from build123d import *

# Parameters (mm, degrees)
SKETCH_1_W            = 42.6
SKETCH_1_H            = 42.6
EXTRUDE_1_DEPTH       = 4
SKETCH_2_R            = 13
CUT_EXTRUDE_1_DEPTH   = 6
FILLET_1_R            = 10
SKETCH_3_W            = 4
SKETCH_3_H            = 22.6
EXTRUDE_2_DEPTH       = 34.5
FILLET_2_R            = 10
SKETCH_4_W            = 12
SKETCH_4_H            = 22.6
EXTRUDE_3_DEPTH       = 6
FILLET_3_R            = 5
FILLET_4_R            = 1
CHAMFER_3_SIZE        = 1
SKETCH_5_R            = 2.5
CUT_EXTRUDE_2_DEPTH   = 56.092921505
CHAMFER_START         = -9.101924
CHAMFER_4_DEPTH       = 6.602294476
CHAMFER_START_2       = 2.5000001
CHAMFER_4_2_DEPTH     = 6.6019239
CHAMFER_START_3       = -2.499629524
CHAMFER_4_3_DEPTH     = 4.999629624
CHAMFER_START_4       = -11.3
CHAMFER_4_4_DEPTH     = 2.198076
CHAMFER_START_5       = 9.101924
CHAMFER_4_5_DEPTH     = 2.198076
CHAMFER_START_6       = 16.5
CHAMFER_4_6_OUTLINE_R = 2.5
CHAMFER_4_6_DEPTH     = 12
SKETCH_6_R            = 4.2
CUT_EXTRUDE_5_DEPTH   = 28


with BuildPart() as part:
    # Эскиз1 → Бобышка-Вытянуть1 (new body)
    with BuildSketch(Plane(origin=(0, 0, 0), x_dir=(1, 0, 0), z_dir=(0, 1, 0))):
        Rectangle(SKETCH_1_W, SKETCH_1_H)
    extrude(amount=EXTRUDE_1_DEPTH)

    # Эскиз2 → Вырез-Вытянуть1 (cut)
    with BuildSketch(Plane(origin=(0, 4, 0), x_dir=(1, 0, 0), z_dir=(0, 1, 0))):
        with Locations(Location((0, 0, 0), (0, 0, 270))):
            Circle(SKETCH_2_R)
    extrude(amount=-CUT_EXTRUDE_1_DEPTH, mode=Mode.SUBTRACT)

    # Скругление1
    fillet_1_edges = [part.edges().sort_by_distance(p)[0] for p in [
        (21.3, 2, 21.3),
        (-21.3, 2, 21.3),
        (-21.3, 2, -21.3),
        (21.3, 2, -21.3),
    ]]
    fillet(fillet_1_edges, radius=FILLET_1_R)

    # Эскиз3 → Бобышка-Вытянуть2 (add)
    with BuildSketch(Plane(origin=(0, 0, 0), x_dir=(1, 0, 0), z_dir=(0, 1, 0))):
        with Locations((-23.3, 0)):
            Rectangle(SKETCH_3_W, SKETCH_3_H)
        with Locations((23.3, 0)):
            Rectangle(SKETCH_3_W, SKETCH_3_H)
    extrude(amount=EXTRUDE_2_DEPTH)

    # Скругление2
    # the kernel refuses this fillet: 10 mm, written as the material it adds along each edge
    with BuildSketch(Plane(origin=(21.3, 0, -11.3), x_dir=(-0.23904572186687842, 0, -0.9710083124552246), z_dir=(0, 1, 0)), Plane(origin=(-21.3, 0, 11.3), x_dir=(0.2390457218668792, 0, 0.9710083124552243), z_dir=(0, 1, 0))) as fillet_2_piece_1:
        with BuildLine():
            CenterArc((7.171371656, -9.710083125), FILLET_2_R, 103.83022495, 40.535802111)
            Line((-0.956182887, -3.88403325), (0, 0))
            ThreePointArc((0, 0), (2.390457219, -0.289916875), (4.780914437, 0))
        make_face()
    extrude(amount=4)
    with BuildSketch(Plane(origin=(-21.3, 0, -11.3), x_dir=(0.23904572186687842, 0, -0.9710083124552246), z_dir=(0, 1, 0)), Plane(origin=(21.3, 0, 11.3), x_dir=(-0.2390457218668792, 0, 0.9710083124552243), z_dir=(0, 1, 0))) as fillet_2_piece_2:
        with BuildLine():
            CenterArc((7.171371656, 9.710083125), FILLET_2_R, 215.633972939, 40.535802111)
            Line((-0.956182887, 3.88403325), (0, 0))
            ThreePointArc((0, 0), (2.390457219, 0.289916875), (4.780914437, 0))
        make_face()
    extrude(amount=4)

    # Эскиз4 → Бобышка-Вытянуть3 (add)
    with BuildSketch(Plane(origin=(0, 34.5, 0), x_dir=(1, 0, 0), z_dir=(0, 1, 0))):
        with Locations((-31.3, 0)):
            Rectangle(SKETCH_4_W, SKETCH_4_H)
        with Locations((31.3, 0)):
            Rectangle(SKETCH_4_W, SKETCH_4_H)
    extrude(amount=-EXTRUDE_3_DEPTH)

    # Скругление3
    fillet_3_edges = [part.edges().sort_by_distance(p)[0] for p in [
        (37.3, 31.5, -11.3),
        (37.3, 31.5, 11.3),
        (-37.3, 31.5, 11.3),
        (-37.3, 31.5, -11.3),
    ]]
    fillet(fillet_3_edges, radius=FILLET_3_R)

    # Скругление4
    fillet_4_edges = [part.edges().sort_by_distance(p)[0] for p in [
        (21.3, 19.25, -11.3),
        (21.3, 19.25, 11.3),
        (21.3, 34.5, 0),
        (-21.3, 19.25, 11.3),
        (-21.3, 19.25, -11.3),
        (-21.3, 34.5, 0),
    ]]
    fillet(fillet_4_edges, radius=FILLET_4_R)

    # Фаска3
    chamfer_3_edges = [part.edges().sort_by_distance(p)[0] for p in [
        (0, 0, -13),
        (0, 0, 21.3),
        (0, 0, -21.3),
        (16.475757114, 0, -19.856374133),
        (-16.475757114, 0, 19.856374133),
        (25.3, 0, 0),
        (-25.3, 0, 0),
        (-16.475757114, 0, -19.856374133),
        (16.475757114, 0, 19.856374133),
        (22.313691772, 0, -13.16154043),
        (-22.313691772, 0, -13.16154043),
        (-22.313691772, 0, 13.16154043),
        (22.313691772, 0, 13.16154043),
    ]]
    chamfer(chamfer_3_edges, length=CHAMFER_3_SIZE)

    # Эскиз5 → Вырез-Вытянуть2 (cut, through all)
    with BuildSketch(Plane(origin=(0, 34.5, 0), x_dir=(1, 0, 0), z_dir=(0, 1, 0))):
        with Locations(Location((30, 0, 0), (0, 0, 270))):
            Circle(SKETCH_5_R)
        with Locations(Location((-30, 0, 0), (0, 0, 90))):
            Circle(SKETCH_5_R)
    extrude(amount=-CUT_EXTRUDE_2_DEPTH, mode=Mode.SUBTRACT)

    # Фаска4: read off the stored shape, not the designer's step
    # Фаска4 outline → Фаска4 (add)
    with BuildSketch(Plane.XY.offset(CHAMFER_START)):
        Polygon((-37.3, 28.5), (-25.3, 16.5), (-25.3, 28.5), align=None)
        Polygon((25.3, 28.5), (25.3, 16.5), (37.3, 28.5), align=None)
    extrude(amount=CHAMFER_4_DEPTH)

    # Chamfer 4 2 outline → Chamfer 4 2 (add)
    with BuildSketch(Plane.XY.offset(CHAMFER_START_2)):
        Polygon((-37.3, 28.5), (-25.3, 16.5), (-25.3, 28.5), align=None)
        Polygon((25.3, 28.5), (25.3, 16.5), (37.3, 28.5), align=None)
    extrude(amount=CHAMFER_4_2_DEPTH)

    # Chamfer 4 3 outline → Chamfer 4 3 (add)
    with BuildSketch(Plane.XY.offset(CHAMFER_START_3)):
        Polygon((-37.3, 28.5), (-25.3, 16.5), (-25.3, 28.5), align=None)
        Polygon((25.3, 28.5), (25.3, 16.5), (37.3, 28.5), align=None)
    extrude(amount=CHAMFER_4_3_DEPTH)

    # Chamfer 4 4 outline → Chamfer 4 4 (add)
    with BuildSketch(Plane.XY.offset(CHAMFER_START_4)):
        Polygon((-37.3, 28.5), (-25.3, 16.5), (-25.3, 28.5), align=None)
        Polygon((25.3, 28.5), (25.3, 16.5), (37.3, 28.5), align=None)
    extrude(amount=CHAMFER_4_4_DEPTH)

    # Chamfer 4 5 outline → Chamfer 4 5 (add)
    with BuildSketch(Plane.XY.offset(CHAMFER_START_5)):
        Polygon((-37.3, 28.5), (-25.3, 16.5), (-25.3, 28.5), align=None)
        Polygon((25.3, 28.5), (25.3, 16.5), (37.3, 28.5), align=None)
    extrude(amount=CHAMFER_4_5_DEPTH)

    # Chamfer 4 6 outline → Chamfer 4 6 (cut)
    with BuildSketch(Plane(origin=(0, 0, 0), x_dir=(1, 0, 0), z_dir=(0, 1, 0)).offset(CHAMFER_START_6)):
        with BuildLine():
            Line((37.299999999, -11.3), (37.3, -6.3))
            ThreePointArc((37.3, -6.3), (35.835533906, -9.835533906), (32.3, -11.3))
            Line((32.3, -11.3), (37.299999999, -11.3))
        make_face()
        with BuildLine():
            ThreePointArc((32.3, 11.3), (35.835533906, 9.835533906), (37.3, 6.3))
            Line((37.3, 6.3), (37.299999999, 11.3))
            Line((37.299999999, 11.3), (32.3, 11.3))
        make_face()
        with BuildLine():
            Line((-37.3, -11.3), (-32.3, -11.3))
            ThreePointArc((-32.3, -11.3), (-35.835533906, -9.835533906), (-37.3, -6.3))
            Line((-37.3, -6.3), (-37.3, -11.3))
        make_face()
        with BuildLine():
            ThreePointArc((-37.3, 6.3), (-35.835533906, 9.835533906), (-32.3, 11.3))
            Line((-32.3, 11.3), (-37.3, 11.3))
            Line((-37.3, 11.3), (-37.3, 6.3))
        make_face()
        with Locations((-30, 0)):
            Circle(CHAMFER_4_6_OUTLINE_R)
        with Locations((30, 0)):
            Circle(CHAMFER_4_6_OUTLINE_R)
    extrude(amount=CHAMFER_4_6_DEPTH, mode=Mode.SUBTRACT)

    # Эскиз6 → Вырез-Вытянуть5 (cut)
    with BuildSketch(Plane.XZ):
        with Locations(Location((30, 0, 0), (0, 0, 270))):
            Circle(SKETCH_6_R)
        with Locations((-30, 0)):
            Circle(SKETCH_6_R)
    extrude(amount=-CUT_EXTRUDE_5_DEPTH, mode=Mode.SUBTRACT)

    # Фаска5
    # the kernel refuses this chamfer: 2 mm, written as the material it takes off along each edge
    with BuildSketch(Plane(origin=(30, 28, 0), x_dir=(1, 0, 0), z_dir=(0, 0, -1))) as chamfer_5_piece_1_section:
        with BuildLine():
            Line((4.556568542, 0.056568542), (2.443431458, -2.056568542))
            Line((2.443431458, -2.056568542), (2.403431458, -2.056568542))
            ThreePointArc((2.403431458, -2.056568542), (2.46, -1.028284271), (2.46, 0))
            Line((2.46, 0), (2.5, 0.04))
            ThreePointArc((2.5, 0.04), (3.528284271, 0.04), (4.556568542, 0.096568542))
            Line((4.556568542, 0.096568542), (4.556568542, 0.056568542))
        make_face()
    chamfer_5_piece_1 = revolve(axis=Axis((30, 28, 0), (0, -1, 0)), mode=Mode.PRIVATE)
    chamfer_5_piece_1 = chamfer_5_piece_1 & Plane(origin=(30, 28, 0), x_dir=(0, 0, -1), z_dir=(0, -1, 0)) * Cylinder(4.2, 19, mode=Mode.PRIVATE)
    add(chamfer_5_piece_1, mode=Mode.SUBTRACT)
    with BuildSketch(Plane(origin=(-30, 28, 0), x_dir=(1, 0, 0), z_dir=(0, 0, -1))) as chamfer_5_piece_2_section:
        with BuildLine():
            Line((2.443431458, -2.056568542), (4.556568542, 0.056568542))
            Line((4.556568542, 0.056568542), (4.556568542, 0.096568542))
            ThreePointArc((4.556568542, 0.096568542), (3.528284271, 0.04), (2.5, 0.04))
            Line((2.5, 0.04), (2.46, 0))
            ThreePointArc((2.46, 0), (2.46, -1.028284271), (2.403431458, -2.056568542))
            Line((2.403431458, -2.056568542), (2.443431458, -2.056568542))
        make_face()
    chamfer_5_piece_2 = revolve(axis=Axis((-30, 28, 0), (0, -1, 0)), mode=Mode.PRIVATE)
    chamfer_5_piece_2 = chamfer_5_piece_2 & Plane(origin=(-30, 28, 0), x_dir=(1, 0, 0), z_dir=(0, -1, 0)) * Cylinder(4.2, 19, mode=Mode.PRIVATE)
    add(chamfer_5_piece_2, mode=Mode.SUBTRACT)


solid = part.part
Part model, mm, in its own coordinate system. A direction names the side the tool comes from. Round coordinates to 2 decimals unless told otherwise and drop trailing zeros. Loops run counter-clockwise (first coordinate to the right, second up) from the corner with the lowest first, then second, coordinate; pieces in that order, holes last. Notation, with made-up numbers: (43.25, 53.25) - (57.25, 53.25) arc R15 cw to (57.25, 62.25) - close; hole circle Ø7 at (33.5, -33.5). An arc over 180 degrees is marked (long way). Answer as a JSON object with one key per item and string values.
Item 1: Tool access for faces 1 (the face through (25.3, 9, 0)), 2 (the face through (-25.3, 9, 0)), 3 (the face through (-25.994, 23.826, 1.262)), 4 (the face through (-26, 23, 11.3)), 5 (the face through (21.3, 19, 0)): list every direction of +Z, -Z, +X, -X, +Y, -Y with a clear straight run to the whole face (end or side of a thin tool).
Output:
{"face 1": "+Z, -Z, +X, -Y", "face 2": "+Z, -Z, -X, -Y", "face 3": "-Y", "face 4": "+Z, +X, -X, +Y", "face 5": "+Z, -Z, +Y"}
Item 2: Pin check, flat tips, straight feed: pin 1 (12 mm diameter, centred on x = 16.5, y = 11.5, fed in from +Z); pin 2 (8 mm diameter, centred on x = 25.5, y = 8.5, fed in from -Z); pin 3 (6 mm diameter, centred on x = -30, z = 0, fed in from -Y). Stop position of each tip, or through.
Output:
{"pin 1": "z = 11.3", "pin 2": "z = -11.3", "pin 3": "y = 29.5"}
Item 3: Pull direction Z, two halves, no side cores. Call faces 6 (the face through (-27.51, 29.89, 0.78)), 7 (the face through (30, 34.5, -3)), 8 (the face through (-26, 23, -11.3)): pulls with the +Z half, pulls with the -Z half, needs draft (parallel to the pull), parting line crosses it, or undercut.
Output:
{"face 6": "undercut", "face 7": "needs draft", "face 8": "pulls with the -Z half"}
Item 4: Wall check: L1, parallel to X at y = 9.5, z = -5; L2, parallel to X at y = 2.5, z = 0; L3, parallel to Z at x = 30, y = 32. Give the ranges that are in metal, low to high.
Output:
{"L1": "-25.3 to -21.3, 21.3 to 25.3", "L2": "-25.3 to -13, 13 to 25.3", "L3": "-11.3 to -2.5, 2.5 to 11.3"}
Item 5: Band-saw the part on B-B on y = 13. List the corners of the cut face in (x, z).
Output:
{"outline": "(-25.3, -11.3) - (-22.3, -11.3) arc R1 ccw to (-21.3, -10.3) - (-21.3, 10.3) arc R1 ccw to (-22.3, 11.3) - (-25.3, 11.3) - close; (21.3, -10.3) arc R1 ccw to (22.3, -11.3) - (25.3, -11.3) - (25.3, 11.3) - (22.3, 11.3) arc R1 ccw to (21.3, 10.3) - close"}
Item 6: Band-saw the part on A-A on y = 31.5. List the corners of the cut face in (x, z), plus the area to 3 significant figures.
Output:
{"outline": "(-37.3, -6.3) arc R5 ccw to (-32.3, -11.3) - (-22.3, -11.3) arc R1 ccw to (-21.3, -10.3) - (-21.3, 10.3) arc R1 ccw to (-22.3, 11.3) - (-32.3, 11.3) arc R5 ccw to (-37.3, 6.3) - close; (21.3, -10.3) arc R1 ccw to (22.3, -11.3) - (32.3, -11.3) arc R5 ccw to (37.3, -6.3) - (37.3, 6.3) arc R5 ccw to (32.3, 11.3) - (22.3, 11.3) arc R1 ccw to (21.3, 10.3) - close; hole circle Ø5 at (-30, 0); hole circle Ø5 at (30, 0)", "area": "662 mm2"}
Item 7: Band-saw the part on D-D on z = 0. State how many separate pieces and enclosed holes the cut face has, plus the area to 3 significant figures.
Output:
{"separate pieces": "4", "enclosed holes": "0", "area": "441 mm2"}
Item 8: Band-saw the part on C-C on x = 0. List the corners of the cut face in (y, z).
Output:
{"outline": "(0, -20.3) - (1, -21.3) - (4, -21.3) - (4, -13) - (1, -13) - (0, -14) - close; (0, 14) - (1, 13) - (4, 13) - (4, 21.3) - (1, 21.3) - (0, 20.3) - close"}
